Geometry: final body of the model. Coordinates: model frame, mm. Face numbers are marked on the shaded views. Coordinates: 2 decimals unless noted, no trailing zeros. Write each loop counter-clockwise with the first axis right and the second up, starting at its lowest first coordinate (ties: lowest second). Pieces come first, ordered by that corner, then holes. Notation, with made-up numbers: (-27, -17) - (23, -17) arc R19 ccw to (23, 17) - close; hole circle Ø8 at (47.25, 86.5). An arc over 180 degrees is marked (long way). Put each result on its own line as item: value.
```python
from build123d import *

# Parameters (mm, degrees)
F0_W     = 10
F0_H     = 5
F4_DEPTH = 5
F6_DEPTH = 5
F7_R     = 1
F8_R     = 1


with BuildPart() as f2:
    # F2: sweep along a path in F1
    with BuildLine(Plane.XY) as f2_path:
        Line((0, 0), (0, 45))
        ThreePointArc((0, 45), (1.4644660941, 48.5355339059), (5, 50))
        Line((5, 50), (20, 50))
    # F0 (on Front) → F2 (sweep)
    with BuildSketch(Plane.XZ):
        Rectangle(F0_W, F0_H)
    sweep(path=f2_path.line)

    # F3 (on face) → F4 (join, through all)
    with BuildSketch(Plane.XY.offset(2.5)):
        Polygon((0, -12.0238676125), (6.5331561742, -8.2519481366), (6.5331561742, -0.708109185), (0, 3.0638102908), (-6.5331561742, -0.708109185), (-6.5331561742, -8.2519481366), align=None)
    extrude(amount=-F4_DEPTH)

    # F5 (on face) → F6 (cut, through all)
    with BuildSketch(Plane.XY.offset(2.5)):
        Polygon((0, -12.0238676125), (3, -10.2918168049), (3, -6.8277151897), (0, -5.0956643822), (-3, -6.8277151897), (-3, -10.2918168049), align=None)
    extrude(amount=-F6_DEPTH, mode=Mode.SUBTRACT)

    # F7
    f7_edges = [f2.edges().sort_by_distance(p)[0] for p in [
        (20, 55, 0),
        (20, 45, 0),
        (5, 45, 0),
    ]]
    fillet(f7_edges, radius=F7_R)

    # F8
    f8_edges = [f2.edges().sort_by_distance(p)[0] for p in [
        (20, 50, 2.5),
        (20, 50, -2.5),
    ]]
    fillet(f8_edges, radius=F8_R)


solid = f2.part
```
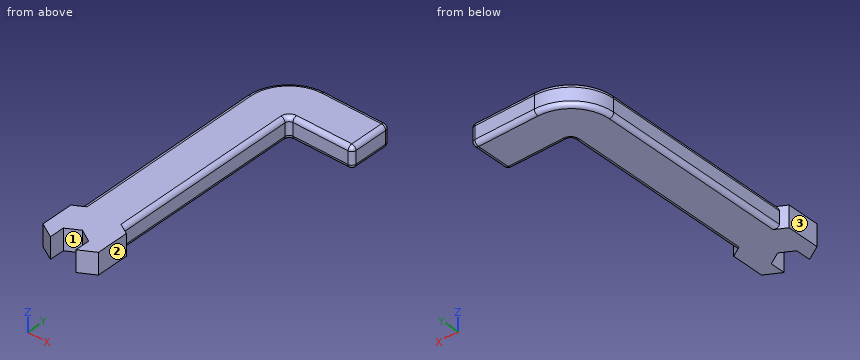
1. Section query A-A (z = 0.75). Return loops of the section in (x, y).
Answer below:
outline: (-6.53, -8.25) - (-3, -10.29) - (-3, -6.83) - (0, -5.1) - (3, -6.83) - (3, -10.29) - (6.53, -8.25) - (6.53, -0.71) - (5, 0.18) - (5, 44) arc R1 cw to (6, 45) - (19, 45) arc R1 ccw to (20, 46) - (20, 54) arc R1 ccw to (19, 55) - (5, 55) arc R10 ccw to (-5, 45) - (-5, 0.18) - (-6.53, -0.71) - close
2. Mould query, pull axis X, two halves, no side actions, for the marked faces 1, 2 and 3. Classes: +X half, -X half, draft (parallel to the pull), parting line (faces both ways), or undercut.
Answer below:
face 1: undercut
face 2: +X half
face 3: -X half
3. Pin query (flat end, axial travel): pin 1 Ø2 at (x, z) = (6.5, 0.5) entering from -Y; pin 2 Ø0.9 at (y, z) = (16.5, 0) entering from -X. Return the tip coordinate at first contact, or that it passes through.
Answer below:
pin 1: stops at y = -8.85
pin 2: stops at x = -5
4. Ray query, probe 1 along X at (y, z) = (-8, 2.1); probe 2 along X at (y, z) = (-3, -0.55); probe 3 along Y at (x, z) = (12.75, -1.25). Return the intervals inside material, ascending. Write a range as from..to.
Answer below:
probe 1: x = -6.53..-3, 3..6.53
probe 2: x = -6.53..6.53
probe 3: y = 45..55
5. Section query B-B (x = 13). Return loops of the section in (y, z), then the cut area to 3 significant figures.
Answer below:
outline: (45, -1.5) arc R1 ccw to (46, -2.5) - (54, -2.5) arc R1 ccw to (55, -1.5) - (55, 1.5) arc R1 ccw to (54, 2.5) - (46, 2.5) arc R1 ccw to (45, 1.5) - close
area: 49.1 mm²
6. Section query C-C (y = 24.5). Return loops of the section in (x, z).
Answer below:
outline: (-5, -1.5) arc R1 ccw to (-4, -2.5) - (4, -2.5) arc R1 ccw to (5, -1.5) - (5, 1.5) arc R1 ccw to (4, 2.5) - (-4, 2.5) arc R1 ccw to (-5, 1.5) - close
